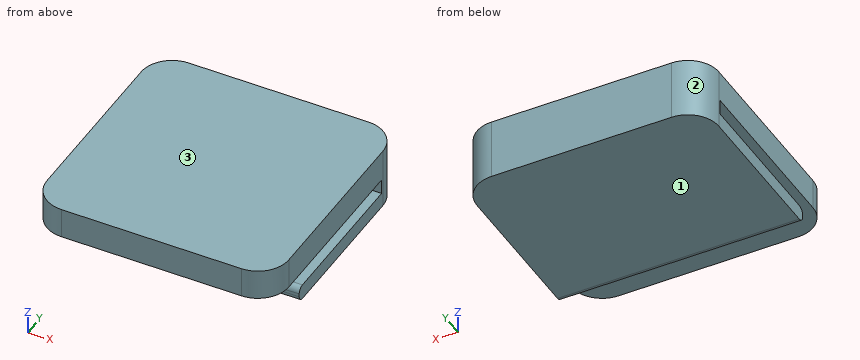
```python
from build123d import *

# Parameters (mm, degrees)
F0_W     = 39.717194
F0_H     = 39.141584
F1_DEPTH = 5
F2_W     = 39.717194
F2_H     = 5.46831
F3_DEPTH = 5
F4_W     = 39.717194
F4_H     = 2.5
F5_DEPTH = 25.4
F6_R     = 5.08
F7_R     = 1


with BuildPart() as f1:
    # F0 (on Top) → F1 (new body)
    with BuildSketch(Plane.XY):
        Rectangle(F0_W, F0_H)
    extrude(amount=F1_DEPTH)

    # F2 (on face) → F3 (join)
    with BuildSketch(Plane(origin=(0, 0, 0), x_dir=(1, 0, 0), z_dir=(0, 0, -1))):
        with Locations((0, -16.836637)):
            Rectangle(F2_W, F2_H)
    extrude(amount=F3_DEPTH)

    # F4 (on face) → F5 (join)
    with BuildSketch(Plane.XZ.offset(-14.102482)):
        with Locations((0, -3.75)):
            Rectangle(F4_W, F4_H)
    extrude(amount=F5_DEPTH)

    # F6
    f6_edges = [f1.edges().sort_by_distance(p)[0] for p in [
        (19.858597, 19.570792, 0),
        (19.858597, -19.570792, 2.5),
        (-19.858597, 19.570792, 0),
        (-19.858597, -19.570792, 2.5),
    ]]
    fillet(f6_edges, radius=F6_R)

    # F7
    f7_edges = [f1.edges().sort_by_distance(p)[0] for p in [
        (0, -11.297518, -5),
        (0, -11.297518, -2.5),
    ]]
    fillet(f7_edges, radius=F7_R)


solid = f1.part
```
Work out the finished part from the listing and answer in its coordinate system (mm). Face numbers are marked on the shaded views. Give positions to 0.01 mm unless a question says otherwise; leave off trailing zeros. Loops run counter-clockwise (first coordinate to the right, second up) from the corner with the lowest first, then second, coordinate; pieces in that order, holes last. Notation, with made-up numbers: M -14.5,42.5 L 15.5,42.5 A12 cw 15.5,48.5 Z; hole C 22.5,-15 d6. An arc over 180 degrees is marked long. One line per item, written item: value. Start each with the question number.
1. Determine the mould class of the marked faces 1, 2 and 3 for opening direction Z: released by +Z, released by -Z, zero draft, split by the parting line, or undercut.
2. Each of these flat-tipped pins is pushed along its axis until it touches: P1, Ø0.8, axis at x = 2.5, z = -0.5, coming from the -Y side; P2, Ø1, axis at x = 12, y = -11.5, coming from the -Z side. Where does it stop, or does it pass through?
3. Find section C-C (z = -1.25). Give the vertices of the cut face in (x, y).
4. Find the intervals of material crossed by probe 1 along Z at (x, y) = (-4, 10); probe 2 along Z at (x, y) = (3, -11.5); probe 3 along Y at (x, z) = (-13.5, -3.75), in increasing order.
5. Find section B-B (x = -12). Give the vertices of the cut face in (y, z), and give its area (3 significant figures).
6. Find section D-D (y = -16). Give the vertices of the cut face in (x, z), and give its area (3 significant figures).
7. Find section A-A (y = 5). Give the vertices of the cut face in (x, z).
Reported:
1. face 1: released by -Z
1. face 2: zero draft
1. face 3: released by +Z
2. P1: stops at y = 14.1
2. P2: stops at z = -4.71
3. outline: M -19.86,14.1 L 19.86,14.1 L 19.86,14.49 A5.08 ccw 14.78,19.57 L -14.78,19.57 A5.08 ccw -19.86,14.49 Z
4. probe 1: z = -5 to -2.5, 0 to 5
4. probe 2: z = 0 to 5
4. probe 3: y = -11.3 to 19.57
5. outline: M -19.57,0 L 14.1,0 L 14.1,-2.5 L -10.3,-2.5 A1 ccw -11.3,-3.5 L -11.3,-4 A1 ccw -10.3,-5 L 19.57,-5 L 19.57,5 L -19.57,5 Z
5. area: 286 mm²
6. outline: M -19.63,0 L 19.63,0 L 19.63,5 L -19.63,5 Z
6. area: 196 mm²
7. outline: M -19.86,-5 L 19.86,-5 L 19.86,-2.5 L -19.86,-2.5 Z; M -19.86,0 L 19.86,0 L 19.86,5 L -19.86,5 Z
